from build123d import *

# Parameters (mm, degrees)
SKETCH_1_R      = 4
EXTRUDE_1_DEPTH = 2.5
EXTRUDE_2_DEPTH = 3


with BuildPart() as part:
    # 草图1 → 凸台-拉伸1 (new body)
    with BuildSketch(Plane(origin=(0, 0, 0), x_dir=(1, 0, 0), z_dir=(0, 1, 0))):
        with Locations(Location((0, 0, 0), (0, 0, 270))):
            Circle(SKETCH_1_R)
        Polygon((0, 3.0022214), (-2.6, 1.5011107), (-2.6, -1.5011107), (0, -3.0022214), (2.6, -1.5011107), (2.6, 1.5011107), align=None, mode=Mode.SUBTRACT)
    extrude(amount=EXTRUDE_1_DEPTH)

    # 草图2 → 凸台-拉伸2 (add)
    with BuildSketch(Plane(origin=(0, 2.5, 0), x_dir=(1, 0, 0), z_dir=(0, 1, 0))):
        with BuildLine():
            Line((4, 0), (4, -20.83484861))
            ThreePointArc((4, -20.83484861), (0, -40), (-4, -20.83484861))
            Line((-4, -20.83484861), (-4, 0))
            ThreePointArc((-4, 0), (0, 4), (4, 0))
        make_face()
    extrude(amount=EXTRUDE_2_DEPTH)


solid = part.part
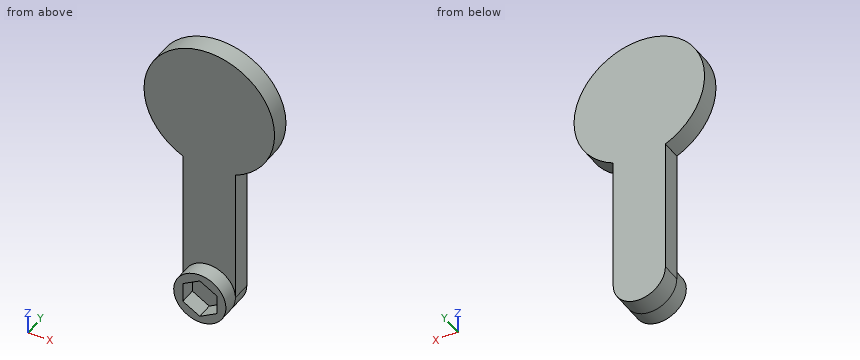
Work out the finished part from the listing and answer in its coordinate system (mm). Give positions to 0.01 mm unless a question says otherwise; leave off trailing zeros. Loops run counter-clockwise (first coordinate to the right, second up) from the corner with the lowest first, then second, coordinate; pieces in that order, holes last. Notation, with made-up numbers: (82, 54) -> (118, 54) arc R18 ccw to (118, 80) -> close; hole circle Ø7 at (11, 86). An arc over 180 degrees is marked (long way). Use a Markdown table: item, result. Add a question column.
1) Each of these flat-tipped pins is pushed along its axis until it touches: P1, Ø4, axis at x = 2, z = 29, coming from the -Y side; P2, Ø3, axis at y = 3.5, z = 16, coming from the +X side; P3, Ø3, axis at y = 1, z = 0.5, coming from the -X side. Where does it stop, or does it pass through?
2) The part is cut by section C-C, the plane z = -0.5. Determine the outline of the cut face in (x, y).
3) The part is cut by section A-A, the plane y = 1.55. Determine the outline of the cut face in (x, z).
4) Consider line 1 along Y through (x, z) = (-8.75, 26); line 2 along X through (y, z) = (2.85, 3); line 3 along X through (y, z) = (0.9, -1). Determine where each line is inside the solid, lowest interval first.
5) The part is cut by section D-D, the plane y = 4.1. Determine the outline of the cut face in (x, z).
6) The part is cut by section B-B, the plane x = -6. Determine the outline of the cut face in (y, z), plus the area to 3 significant figures.
Reported:
| question | item | result |
|---|---|---|
| 1 | P1 | stops at y = 2.5 |
| 1 | P2 | stops at x = 4 |
| 1 | P3 | stops at x = -4 |
| 2 | outline | (-3.97, 0) -> (-2.6, 0) -> (-2.6, 2.5) -> (2.6, 2.5) -> (2.6, 0) -> (3.97, 0) -> (3.97, 5.5) -> (-3.97, 5.5) -> close |
| 3 | outline | circle Ø8 at (0, 0); hole (-2.6, -1.5) -> (0, -3) -> (2.6, -1.5) -> (2.6, 1.5) -> (0, 3) -> (-2.6, 1.5) -> close |
| 4 | line 1 | y = 2.5 to 5.5 |
| 4 | line 2 | x = -4 to 4 |
| 4 | line 3 | x = -3.87 to -2.6, 2.6 to 3.87 |
| 5 | outline | (-4, 0) arc R4 ccw to (4, 0) -> (4, 20.83) arc R10 ccw (long way) to (-4, 20.83) -> close |
| 6 | outline | (2.5, 22) -> (5.5, 22) -> (5.5, 38) -> (2.5, 38) -> close |
| 6 | area | 48.0 mm^2 |
